from build123d import *

# Parameters (mm, degrees)
BOSS_EXTRUDE1_DEPTH  = 6
FILLET1_R            = 5
SKETCH2_R            = 2.25
SKETCH2_R_2          = 1.6
CUT_EXTRUDE1_DEPTH   = 117.773284616
FILLET1_OF_MIRROR1_R = 5


with BuildPart() as part:
    # Sketch1 → Boss-Extrude1 (new body)
    with BuildSketch(Plane(origin=(0, 0, 0), x_dir=(1, 0, 0), z_dir=(0, 1, 0))):
        Polygon((0, 0), (-85, 0), (-85, 60), (-100, 60), (-100, -15), (0, -15), align=None)
    boss_extrude1 = extrude(amount=BOSS_EXTRUDE1_DEPTH)

    # Fillet1
    fillet1_edges = [part.edges().sort_by_distance(p)[0] for p in [
        (-100, 3, 15),
        (-100, 3, -60),
        (-85, 3, -60),
        (-85, 3, 0),
    ]]
    fillet(fillet1_edges, radius=FILLET1_R)

    # Sketch2 → Cut-Extrude1 (cut, through all)
    with BuildSketch(Plane(origin=(0, 6, 0), x_dir=(1, 0, 0), z_dir=(0, 1, 0))):
        with Locations(Location((-15, -7.5, 0), (0, 0, 270))):
            Circle(SKETCH2_R)
        with Locations(Location((-80, -7.5, 0), (0, 0, 270))):
            Circle(SKETCH2_R_2)
    cut_extrude1 = extrude(amount=-CUT_EXTRUDE1_DEPTH, mode=Mode.SUBTRACT)

    # Mirror1: Boss-Extrude1, Cut-Extrude1 across plane
    add(boss_extrude1.mirror(Plane(origin=(0, 0, 0), x_dir=(0, 0, 1), z_dir=(1, 0, 0))))
    add(cut_extrude1.mirror(Plane(origin=(0, 0, 0), x_dir=(0, 0, 1), z_dir=(1, 0, 0))), mode=Mode.SUBTRACT)

    # Fillet1 of Mirror1
    fillet1_of_mirror1_edges = [part.edges().sort_by_distance(p)[0] for p in [
        (100, 3, 15),
        (100, 3, -60),
        (85, 3, -60),
        (85, 3, 0),
    ]]
    fillet(fillet1_of_mirror1_edges, radius=FILLET1_OF_MIRROR1_R)


solid = part.part
Model file for the job. Use its own axes, mm. A direction names the side the tool comes from. Round coordinates to 2 decimals unless told otherwise and drop trailing zeros. Loops run counter-clockwise (first coordinate to the right, second up) from the corner with the lowest first, then second, coordinate; pieces in that order, holes last. Notation, with made-up numbers: (83.5, -28) -> (89.5, -28) arc R26 ccw to (89.5, 3) -> close; hole circle Ø3 at (46.5, 53.25). An arc over 180 degrees is marked (long way). Answer as CSV lines item,"result". Start each with the question number.
1) Slice it at B-B (z = -44). List the corners of the cut face in (x, y), plus the area to 3 significant figures.
2) Tool access for faces 1 (the face through (-85, 3, -30)), 2 (the face through (98, 3, -59)): list every direction of +Z, -Z, +X, -X, +Y, -Y with a clear straight run to the whole face (end or side of a thin tool).
3) Pin check, flat tips, straight feed: P1, Ø3, axis at x = 54, y = 2.5, coming from the -Z side; P2, Ø10, axis at x = 14, z = -8, coming from the +Y side; P3, Ø5, axis at x = -15, z = 7.5, coming from the +Y side. Stop position of each tip, or through.
4) Slice it at A-A (x = 15). List the corners of the cut face in (y, z), plus the area to 3 significant figures.
5) Slice it at D-D (x = -46). List the corners of the cut face in (y, z).
6) Mould opens along Z. For faces 3 (the face through (17.196, 3.042, 7.012)), 4 (the face through (83, 3, -1)), 5 (the face through (1, 0, 2)) say: +Z half, -Z half, draft (parallel to the pull), parting line (faces both ways), or undercut.
7) Probe line 1 along X through (y, z) = (2.25, 7.5); line 2 along Z through (x, y) = (80, 3.6); line 3 along X through (y, z) = (5.1, -31). List the from-to ranges inside material, lowest first.
8) Slice it at C-C (y = 1.2). List the corners of the cut face in (x, z), plus the area to 3 significant figures.
Filled in:
1,outline,"(-100, 0) -> (-85, 0) -> (-85, 6) -> (-100, 6) -> close; (85, 0) -> (100, 0) -> (100, 6) -> (85, 6) -> close"
1,area,"180 mm2"
2,face 1,"-Z, +Y, -Y"
2,face 2,"-Z, +X, +Y, -Y"
3,P1,"stops at z = 0"
3,P2,"passes through"
3,P3,"stops at y = 6"
4,outline,"(0, 0) -> (6, 0) -> (6, 5.25) -> (0, 5.25) -> close; (0, 9.75) -> (6, 9.75) -> (6, 15) -> (0, 15) -> close"
4,area,"63.0 mm2"
5,outline,"(0, 0) -> (6, 0) -> (6, 15) -> (0, 15) -> close"
6,face 3,"undercut"
6,face 4,"-Z half"
6,face 5,"draft"
7,line 1,"x = -100 to -81.6, -78.4 to -17.25, -12.75 to 12.75, 17.25 to 78.4, 81.6 to 100"
7,line 2,"z = 0 to 5.9, 9.1 to 15"
7,line 3,"x = -100 to -85, 85 to 100"
8,outline,"(-100, -55) arc R5 ccw to (-95, -60) -> (-90, -60) arc R5 ccw to (-85, -55) -> (-85, -5) arc R5 cw to (-80, 0) -> (80, 0) arc R5 cw to (85, -5) -> (85, -55) arc R5 ccw to (90, -60) -> (95, -60) arc R5 ccw to (100, -55) -> (100, 10) arc R5 ccw to (95, 15) -> (-95, 15) arc R5 ccw to (-100, 10) -> close; hole circle Ø3.2 at (-80, 7.5); hole circle Ø4.5 at (-15, 7.5); hole circle Ø4.5 at (15, 7.5); hole circle Ø3.2 at (80, 7.5)"
8,area,"4,730 mm2"
